Read the model definition and answer for the solid it produces. Units are mm, in the model's axes. A direction names the side the tool comes from. Round coordinates to 2 decimals unless told otherwise and drop trailing zeros. Order: outer loops, then holes, each group sorted by start corner. A loop starts at its lowest first (then second) coordinate and runs counter-clockwise, first axis right, second up. Notation, with made-up numbers: (-11.75, -26.5) -> (30.25, -26.5) arc R23 cw to (30.25, 11.5) -> close; hole circle Ø1 at (60, 10). An arc over 180 degrees is marked (long way). Use a Markdown table: item, result. Add a question column.
1. Section A-A, the plane x = 0 is taken. Give the vertices of the cut face in (y, z) (3 decimals), then the cut area to 3 significant figures.
2. Consider L1, parallel to Z at x = 16, y = -9; L2, parallel to Y at x = 6, z = 109.5; L3, parallel to Y at x = 5.5, z = 23. Determine where each line is inside the solid, lowest interval first. Write a range as [from, to].
3. The mould has two halves that part along X. Classify faces 3 (the face through (0, -20, 2.54)), 4 (the face through (0, 3.175, 144)), 5 (the face through (18.82, -21, 8)): +X half, -X half, draft (parallel to the pull), parting line (faces both ways), or undercut.
4. Section C-C, the plane z = 121.5 is taken. Give the vertices of the cut face in (x, y), then the cut area to 3 significant figures.
5. Section D-D, the plane x = -8 is taken. Give the vertices of the cut face in (y, z), then the cut area to 3 significant figures.
6. Given pin 1 (5 mm diameter, centred on x = -8.5, z = 60.5, fed in from -Y); pin 2 (4 mm diameter, centred on x = -1.5, y = -31, fed in from +Z); pin 3 (6 mm diameter, centred on y = -6.5, z = 66, fed in from -X), each flat-ended and moving along its own axis, determine where each tip first touches the part or whether it passes through.
7. For faces 1 (the face through (-1.29, -9.82, 80.32)), 2 (the face through (-16.923, 13.644, 7.549)), determine the directions among +Z, -Z, +X, -X, +Y, -Y from which every point of the face is accessible in a straight line to the end or side of a thin tool.
8. Section B-B, the plane y = 0 is taken. Give the vertices of the cut face in (x, z) (3 decimals), then the cut area to 3 significant figures.
Autodesk Inventor part; units mm, degrees
ref_plane "YZ Plane" through (0, 0, 0) normal (1, 0, 0) x (0, 1, 0)
ref_plane "XZ Plane" through (0, 0, 0) normal (0, 1, 0) x (-1, 0, 0)
ref_plane "XY Plane" through (0, 0, 0) normal (0, 0, 1) x (1, 0, 0)
sketch "Sketch1" plane through (0, 0, 0) normal (0, 0, 1) x (1, 0, 0)
  circle A0 centre (0, 0) radius 9.906
  dimension "d0" = 19.812
extrude "Extrusion1" add sketch "Sketch1" along normal blind 149.86
sketch "Sketch2" plane through (0, 0, 149.86) normal (0, 0, 1) x (1, 0, 0)
  circle A0 centre (0, 0) radius 9.906
  circle A1 centre (0, 0) radius 3.175
  line L0 (-3.175, 0) -> (0, 0)
  line L1 (0, 0) -> (0, 3.175)
  line L2 (0, 3.175) -> (-3.175, 3.175)
  line L3 (-3.175, 3.175) -> (-3.175, 0)
  line L4 (-3.175, 3.175) -> (3.175, 3.175)
  line L5 (3.175, 3.175) -> (3.175, -3.175)
  line L6 (3.175, -3.175) -> (-3.175, -3.175)
  line L7 (-3.175, -3.175) -> (-3.175, 3.175)
  dimension "d3" = 6.35
extrude "Extrusion2" cut sketch "Sketch2" against normal blind 12.7 contours A1 L0 L1 | L5 L6 A1 | A1 L4 L5 | L1 L0 A1 | A1 L3 L2 | L6 L7 A1
sketch "Sketch3" plane through (0, 0, 0) normal (0, 0, -1) x (-1, 0, 0)
  circle A0 centre (0, 0) radius 9.906
  line L0 (0, 0) -> (-25.4, 0)
  line L1 (-25.4, 0) -> (-25.4, 25.4)
  line L2 (-25.4, 25.4) -> (0, 25.4)
  line L3 (0, 25.4) -> (0, 0)
  line L4 (-25.4, 25.4) -> (25.4, 25.4)
  line L5 (25.4, 25.4) -> (25.4, -25.4)
  line L6 (25.4, -25.4) -> (-25.4, -25.4)
  line L7 (-25.4, -25.4) -> (-25.4, 25.4)
  dimension "d6" = 25.4
  dimension "d7" = 25.4
  dimension "d8" = 50.8
  dimension "d9" = 50.8
extrude "Extrusion3" add sketch "Sketch3" against normal blind 12.7 contours A0 L3 L4 L5 L6 L7 L0 | L3 L0 A0 | A0 L0 L1 L2 L3 picked at (-6.1942, 2.1674)
sketch "Sketch4" plane through (-25.4, 25.4, 0) normal (0, 1, 0) x (1, 0, 0)
  line L0 (0, -12.7) -> (50.8, -12.7)
  line L1 (50.8, 0) -> (50.8, -12.7)
  line L2 (0, 0) -> (50.8, 0)
  line L3 (0, 0) -> (0, -12.7)
  point P0 (25.4, 0)
extrude "Extrusion4" cut sketch "Sketch4" against normal blind 6.35
sketch "Sketch5" plane through (0, 0, 0) normal (0, 0, -1) x (-1, 0, 0)
  line L0 (25.4, 19.05) -> (-25.4, 19.05)
  line L1 (-25.4, 19.05) -> (-25.4, -25.4)
  line L2 (-25.4, -25.4) -> (25.4, -25.4)
  line L3 (25.4, -25.4) -> (25.4, 19.05)
  line L4 (-25.4, 19.05) -> (25.4, 19.05)
  line L5 (25.4, 19.05) -> (25.4, -31.75)
  line L6 (25.4, -31.75) -> (-25.4, -31.75)
  line L7 (-25.4, -31.75) -> (-25.4, 19.05)
  point P0 (0, 0)
  dimension "d14" = 50.8
extrude "Extrusion5" add sketch "Sketch5" against normal blind 12.7 contours L5 L6 L7 L2
sketch "Sketch7" plane through (0, 0, 12.7) normal (0, 0, 1) x (1, 0, 0)
  line L0 (25.4, 19.05) -> (25.4, -31.75)
  circle A0 centre (0, 0) radius 9.906
  line L1 (0, 9.906) -> (0, 16.6116)
  line L2 (0, 16.6116) -> (-19.7866, 16.6116)
  line L3 (-19.7866, 16.6116) -> (-19.7866, -57.277)
  line L4 (-19.7866, -57.277) -> (0, -57.277)
  line L5 (0, -57.277) -> (0, 16.6116)
  line L6 (-19.7866, 16.6116) -> (19.7866, 16.6116)
  line L7 (19.7866, 16.6116) -> (19.7866, -57.277)
  line L8 (19.7866, -57.277) -> (-19.7866, -57.277)
  line L9 (-19.7866, -57.277) -> (-19.7866, 16.6116)
  dimension "d17" = 6.7056
  dimension "d18" = 19.7866
  dimension "d19" = 73.8886
  dimension "d20" = 39.5732
extrude "Extrusion6" add sketch "Sketch7" against normal blind 50.8 contours A0 L1 L6 L7 L8 L5 | L5 A0 | A0 L5 L4 L3 L2 L1 picked at (-4.6219, 0.7927)
sketch "Sketch8" plane through (0, 0, 0) normal (0, 0, -1) x (-1, 0, 0)
  line L0 (-19.7866, -31.75) -> (-19.7866, 16.6116)
  line L1 (-19.7866, 16.6116) -> (19.7866, 16.6116)
  line L2 (19.7866, 16.6116) -> (19.7866, -31.75)
  line L3 (19.7866, -31.75) -> (25.4, -31.75)
  line L4 (25.4, -31.75) -> (25.4, 19.05)
  line L5 (25.4, 19.05) -> (-25.4, 19.05)
  line L6 (-25.4, 19.05) -> (-25.4, -31.75)
  line L7 (-25.4, -31.75) -> (-19.7866, -31.75)
  point P0 (0, 0)
extrude "Extrusion7" cut sketch "Sketch8" against normal blind 50.8
fillet "Fillet1" radius 6.35 4 edges at (19.7866, 16.6116, -12.7) (-19.7866, 16.6116, -12.7) (19.7866, -57.277, -12.7) (-19.7866, -57.277, -12.7)
sketch "Sketch9" plane through (0, 0, -38.1) normal (0, 0, -1) x (-1, 0, 0)
  arc A0 (13.4366, -57.277) -> (19.7866, -50.927) centre (13.4366, -50.927) ccw
  line L0 (19.7866, 10.2616) -> (19.7866, -50.927)
  arc A1 (19.7866, 10.2616) -> (13.4366, 16.6116) centre (13.4366, 10.2616) ccw
  line L1 (-13.4366, 16.6116) -> (13.4366, 16.6116)
  arc A2 (-13.4366, 16.6116) -> (-19.7866, 10.2616) centre (-13.4366, 10.2616) ccw
  line L2 (-19.7866, -50.927) -> (-19.7866, 10.2616)
  arc A3 (-19.7866, -50.927) -> (-13.4366, -57.277) centre (-13.4366, -50.927) ccw
  line L3 (13.4366, -57.277) -> (-13.4366, -57.277)
  line L4 (0, -9.906) -> (0, 9.906)
  arc A4 (0, 9.906) -> (0, -9.906) centre (0, 0) ccw
extrude "Extrusion8" cut sketch "Sketch9" against normal blind 25.4
sketch "Sketch10" plane through (0, 0, -12.7) normal (0, 0, -1) x (-1, 0, 0)
  arc A0 (0, 9.906) -> (0, -9.906) centre (0, 0) ccw
  line L0 (0, -9.906) -> (0, 9.906)
extrude "Extrusion9" add sketch "Sketch10" against normal blind 25.4
sketch "Sketch11" plane through (0, 0, -12.7) normal (0, 0, -1) x (-1, 0, 0)
  line L0 (19.7866, 10.2616) -> (19.7866, -50.927)
  arc A0 (19.7866, 10.2616) -> (13.4366, 16.6116) centre (13.4366, 10.2616) ccw
  line L1 (-13.4366, 16.6116) -> (13.4366, 16.6116)
  arc A1 (-13.4366, 16.6116) -> (-19.7866, 10.2616) centre (-13.4366, 10.2616) ccw
  line L2 (-19.7866, -50.927) -> (-19.7866, 10.2616)
  arc A2 (-19.7866, -50.927) -> (-13.4366, -57.277) centre (-13.4366, -50.927) ccw
  line L3 (13.4366, -57.277) -> (-13.4366, -57.277)
  arc A3 (13.4366, -57.277) -> (19.7866, -50.927) centre (13.4366, -50.927) ccw
  point P0 (0, 0)
extrude "Extrusion10" cut sketch "Sketch11" against normal blind 12.7
sketch "Sketch12" plane through (0, 0, 0) normal (0, 0, -1) x (-1, 0, 0)
  line L0 (-19.7866, 16.6116) -> (19.7866, 16.6116)
  line L1 (19.7866, 16.6116) -> (19.7866, -57.277)
  line L2 (19.7866, -57.277) -> (-19.7866, -57.277)
  line L3 (-19.7866, -57.277) -> (-19.7866, 16.6116)
  point P0 (0, 0)
extrude "Extrusion11" add sketch "Sketch12" against normal blind 12.7
fillet "Fillet2" radius 7.62 4 edges at (19.7866, 16.6116, 6.35) (-19.7866, 16.6116, 6.35) (-19.7866, -57.277, 6.35) (19.7866, -57.277, 6.35)
sketch "Sketch13" plane through (0, 0, 0) normal (0, 0, -1) x (-1, 0, 0)
  arc A0 (-19.7866, -49.657) -> (-12.1666, -57.277) centre (-12.1666, -49.657) ccw
  line L0 (12.1666, -57.277) -> (-12.1666, -57.277)
  arc A1 (12.1666, -57.277) -> (19.7866, -49.657) centre (12.1666, -49.657) ccw
  line L1 (19.7866, 8.9916) -> (19.7866, -49.657)
  arc A2 (19.7866, 8.9916) -> (12.1666, 16.6116) centre (12.1666, 8.9916) ccw
  line L2 (-12.1666, 16.6116) -> (12.1666, 16.6116)
  arc A3 (-12.1666, 16.6116) -> (-19.7866, 8.9916) centre (-12.1666, 8.9916) ccw
  line L3 (-19.7866, -49.657) -> (-19.7866, 8.9916)
  arc A4 (18.8199, 8.9916) -> (12.1666, 15.6449) centre (12.1666, 8.9916) ccw
  line L4 (18.8199, 8.9916) -> (18.8199, -49.657)
  arc A5 (12.1666, -56.3103) -> (18.8199, -49.657) centre (12.1666, -49.657) ccw
  line L5 (12.1666, -56.3103) -> (-12.1666, -56.3103)
  arc A6 (-18.8199, -49.657) -> (-12.1666, -56.3103) centre (-12.1666, -49.657) ccw
  line L6 (-18.8199, -49.657) -> (-18.8199, 8.9916)
  arc A7 (-12.1666, 15.6449) -> (-18.8199, 8.9916) centre (-12.1666, 8.9916) ccw
  line L7 (-12.1666, 15.6449) -> (12.1666, 15.6449)
  point P0 (0, 0)
extrude "Extrusion12" cut sketch "Sketch13" against normal blind 12.7
sketch "Sketch14" plane through (0, 0, 0) normal (0, 0, -1) x (-1, 0, 0)
  line L0 (12.1666, 15.6449) -> (-12.1666, 15.6449)
  arc A0 (-12.1666, 15.6449) -> (-18.8199, 8.9916) centre (-12.1666, 8.9916) ccw
  line L1 (-18.8199, 8.9916) -> (-18.8199, -49.657)
  arc A1 (-18.8199, -49.657) -> (-12.1666, -56.3103) centre (-12.1666, -49.657) ccw
  line L2 (-12.1666, -56.3103) -> (12.1666, -56.3103)
  arc A2 (12.1666, -56.3103) -> (18.8199, -49.657) centre (12.1666, -49.657) ccw
  line L3 (18.8199, -49.657) -> (18.8199, 8.9916)
  arc A3 (18.8199, 8.9916) -> (12.1666, 15.6449) centre (12.1666, 8.9916) ccw
  point P0 (0, 0)
extrude "Extrusion13" cut sketch "Sketch14" against normal blind 2.54
sketch "Sketch15" plane through (0, 0, 2.54) normal (0, 0, -1) x (-1, 0, 0)
  arc A0 (-12.1666, 15.6449) -> (-18.8199, 8.9916) centre (-12.1666, 8.9916) ccw
  line L0 (-18.8199, -49.657) -> (-18.8199, 8.9916)
  arc A1 (-18.8199, -49.657) -> (-12.1666, -56.3103) centre (-12.1666, -49.657) ccw
  line L1 (12.1666, -56.3103) -> (-12.1666, -56.3103)
  arc A2 (12.1666, -56.3103) -> (18.8199, -49.657) centre (12.1666, -49.657) ccw
  line L2 (18.8199, 8.9916) -> (18.8199, -49.657)
  arc A3 (18.8199, 8.9916) -> (12.1666, 15.6449) centre (12.1666, 8.9916) ccw
  line L3 (-12.1666, 15.6449) -> (12.1666, 15.6449)
  point P0 (0, 0)
properties part number "linac arm2"
Verdict:
| question | item | result |
|---|---|---|
| 1 | outline | (-56.31, 2.54) -> (15.645, 2.54) -> (15.645, 12.7) -> (9.906, 12.7) -> (9.906, 149.86) -> (3.175, 149.86) -> (3.175, 137.16) -> (-3.175, 137.16) -> (-3.175, 149.86) -> (-9.906, 149.86) -> (-9.906, 12.7) -> (-56.31, 12.7) -> close |
| 1 | area | 3,370 mm2 |
| 2 | L1 | z = [2.54, 12.7] |
| 2 | L2 | y = [-7.88, 7.88] |
| 2 | L3 | y = [-8.24, 8.24] |
| 3 | face 3 | draft |
| 3 | face 4 | undercut |
| 3 | face 5 | +X half |
| 4 | outline | circle Ø19.81 at (0, 0) |
| 4 | area | 308 mm2 |
| 5 | outline | (-56.31, 2.54) -> (15.64, 2.54) -> (15.64, 12.7) -> (5.84, 12.7) -> (5.84, 149.86) -> (-5.84, 149.86) -> (-5.84, 12.7) -> (-56.31, 12.7) -> close |
| 5 | area | 2,330 mm2 |
| 6 | pin 1 | stops at y = -7.88 |
| 6 | pin 2 | stops at z = 12.7 |
| 6 | pin 3 | stops at x = -9.27 |
| 7 | face 1 | +Z |
| 7 | face 2 | +Z, -Z, -X, +Y |
| 8 | outline | (-18.82, 2.54) -> (18.82, 2.54) -> (18.82, 12.7) -> (9.906, 12.7) -> (9.906, 149.86) -> (3.175, 149.86) -> (3.175, 137.16) -> (-3.175, 137.16) -> (-3.175, 149.86) -> (-9.906, 149.86) -> (-9.906, 12.7) -> (-18.82, 12.7) -> close |
| 8 | area | 3,020 mm2 |
